Verification items for the finished model (mm, model axes). Round coordinates to 2 decimals unless told otherwise and drop trailing zeros. Write each loop counter-clockwise with the first axis right and the second up, starting at its lowest first coordinate (ties: lowest second). Pieces come first, ordered by that corner, then holes. Notation, with made-up numbers: M 57.25,6.5 L 111.25,6.5 A4 ccw 111.25,11.5 Z; hole C 87.25,-26 d1. An arc over 180 degrees is marked long. One line per item, written item: value. Start each with the question number.
Item 1: Thickness scan on probe 1 along X at (y, z) = (8.25, 110) (3 decimals); probe 2 along Y at (x, z) = (1.05, 114.3). Record the ranges inside material, lowest first. Write a range as from..to.
Item 2: Section check B-B, the plane y = 17.75. Record the cut outline in (x, z) (3 decimals).
Item 3: Section check C-C, the plane z = 73. Record the cut outline in (x, y) (3 decimals).
Item 4: Section check A-A, the plane z = 165.1. Record the cut outline in (x, y) (3 decimals).
Item 5: Gauge pin test, flat ends, axial feed: pin 1 (8 mm diameter, centred on y = 12.7, z = 139.7, fed in from -X); pin 2 (10 mm diameter, centred on x = 12.7, z = 190.5, fed in from +Y) (3 decimals). Record the tip position at first contact, or that the pin passes through.
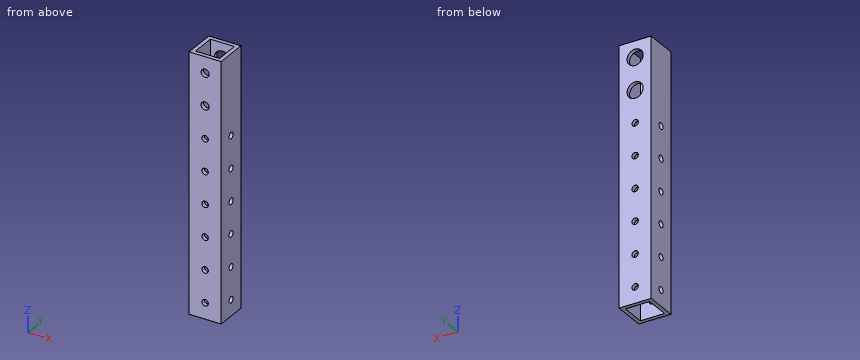
Autodesk Inventor part; units mm, degrees
ref_plane "YZ Plane" through (0, 0, 0) normal (1, 0, 0) x (0, 1, 0)
ref_plane "XZ Plane" through (0, 0, 0) normal (0, 1, 0) x (-1, 0, 0)
ref_plane "XY Plane" through (0, 0, 0) normal (0, 0, 1) x (1, 0, 0)
sketch "Sketch2" plane through (0, 0, 0) normal (0, 0, 1) x (1, 0, 0)
  line L0 (0, 0) -> (25.4, 0)
  line L1 (25.4, 0) -> (25.4, 25.4)
  line L2 (25.4, 25.4) -> (0, 25.4)
  line L3 (0, 25.4) -> (0, 0)
  line L4 (3.175, 22.225) -> (22.225, 22.225)
  line L5 (22.225, 22.225) -> (22.225, 3.175)
  line L6 (22.225, 3.175) -> (3.175, 3.175)
  line L7 (3.175, 3.175) -> (3.175, 22.225)
  dimension "d0" = 25.4
  dimension "d1" = 25.4
  dimension "d2" = 3.175
extrude "Extrusion1" add sketch "Sketch2" along normal blind 203.2
sketch "Sketch5" plane through (0, 0, 0) normal (-1, 0, 0) x (0, 0, 1)
  circle A0 centre (139.7, 12.7) radius 2.54
  line L0 (203.2, 25.4) -> (203.2, 0)
  line L1 (0, 25.4) -> (203.2, 25.4)
  circle A1 centre (114.3, 12.7) radius 2.54
  circle A2 centre (88.9, 12.7) radius 2.54
  circle A3 centre (63.5, 12.7) radius 2.54
  circle A4 centre (38.1, 12.7) radius 2.54
  circle A5 centre (12.7, 12.7) radius 2.54
  point P0 (0, 0)
  point P1 (203.2, 12.7)
  point P2 (203.2, 12.7)
  dimension "d13" = 5.08
  dimension "d15" = 63.5
  dimension "d23" = 25.4
extrude "Extrusion4" cut sketch "Sketch5" against normal through all
sketch "Sketch6" plane through (0, 25.4, 0) normal (0, 1, 0) x (1, 0, 0)
  line L0 (25.4, -203.2) -> (0, -203.2)
  line L1 (0, 0) -> (0, -203.2)
  point P0 (12.7, -190.5)
  dimension "d28" = 12.7
  dimension "d29" = 12.7
hole "Hole1" at (12.7, 25.4, 190.5) direction (0, -1, 0) diameter 6.35 end through all counterbore diameter 12.7 counterbore depth 6.35
pattern_linear "Rectangular Pattern1" count 2 spacing 25.4 along (0, 0, -1) of "Hole1"
sketch "Sketch7" plane through (0, 25.4, 0) normal (0, 1, 0) x (1, 0, 0)
  line L0 (25.4, -203.2) -> (0, -203.2)
  line L1 (0, 0) -> (0, -203.2)
  point P0 (12.7021, -139.7)
  dimension "d40" = 63.5
  dimension "d41" = 12.7021
hole "Hole2" at (12.7021, 25.4, 139.7) direction (0, -1, 0) diameter 5.08 end through all
pattern_linear "Rectangular Pattern2" count 6 spacing 25.4 along (0, 0, -1) of "Hole2"
equation "\"d0\" = d1"
properties part number "testRoboRescue_Chassis_Frame_heightBar" material "Aluminum 6061"
Response values:
1. probe 1: x = 0..3.175, 22.225..25.4
1. probe 2: y = 0..10.16, 15.24..25.4
2. outline: M 0,0 L 3.175,0 L 3.175,203.2 L 0,203.2 Z; M 22.225,0 L 25.4,0 L 25.4,203.2 L 22.225,203.2 Z
3. outline: M 0,0 L 25.4,0 L 25.4,25.4 L 0,25.4 Z; hole M 3.175,3.175 L 22.225,3.175 L 22.225,22.225 L 3.175,22.225 Z
4. outline: M 0,0 L 9.525,0 L 9.525,3.175 L 3.175,3.175 L 3.175,22.225 L 6.35,22.225 L 6.35,25.4 L 0,25.4 Z; M 15.875,0 L 25.4,0 L 25.4,25.4 L 19.05,25.4 L 19.05,22.225 L 22.225,22.225 L 22.225,3.175 L 15.875,3.175 Z
5. pin 1: stops at x = 0
5. pin 2: stops at y = 3.175
